For this review, take the finished solid that the model builds, in its own axes (mm). Coordinates: 2 decimals unless noted, no trailing zeros. Write each loop counter-clockwise with the first axis right and the second up, starting at its lowest first coordinate (ties: lowest second). Pieces come first, ordered by that corner, then holes. Notation, with made-up numbers: (29, 1.5) -> (63, 1.5) arc R17 ccw to (63, 10.5) -> close; hole circle Ø9 at (-36, -14.75). An arc over 180 degrees is marked (long way). One line per item, written item: value. Start each with the question number.
1) Add section D-D (z = -62). State the section outline as (x, y) points.
2) Add section C-C (x = -84.5). State the section outline as (y, z) points, and give its area (3 significant figures).
3) Add section B-B (y = 1.2). State how many separate pieces and enclosed holes the cut face has, and give its area (3 significant figures).
4) Add section A-A (x = -40). State the section outline as (y, z) points.
5) For probe 1 along Z at (x, y) = (0, 1.25); probe 2 along Z at (x, y) = (40, 1.1); probe 3 along X at (y, z) = (0.95, 9.5), list the stretches that pass through material, from the lowest coordinate up. Write a range as from..to.
6) Mouldability with a two-part tool opening along X and no side actions: class faces 1 (the flat face through (-78.233, 1.479, -63.383)), 2 (the cylindrical face through (44.995, 1.521, 6.667)), 3 (the flat face through (77.331, 1.479, -64.285)) as released by +X, released by -X, zero draft, split by the parting line, or undercut.
from build123d import *

# Parameters (mm, degrees)
EXTRUDE1_DEPTH     = 3
SKETCH2_R          = 5
CUT_EXTRUDE1_DEPTH = 4
SKETCH7_R          = 5
CUT_EXTRUDE6_DEPTH = 4
SKETCH8_R          = 2.1
CUT_EXTRUDE7_DEPTH = 4


with BuildPart() as part:
    # Sketch1 → Extrude1 (new body)
    with BuildSketch(Plane(origin=(0, 0, 0), x_dir=(1, 0, 0), z_dir=(0, 1, 0))):
        Polygon((-110, -13.947380088), (-110, 31.616111773), (-45.563491861, 96.052619912), (0, 96.052619912), (45.563491861, 96.052619912), (110, 31.616111773), (110, -13.947380088), align=None)
    extrude(amount=EXTRUDE1_DEPTH)

    # Sketch2 → Cut-Extrude1 (cut, through all)
    with BuildSketch(Plane(origin=(0, 3, 0), x_dir=(-1, 0, 0), z_dir=(0, 1, 0))):
        with Locations((85, 6.447380088)):
            Circle(SKETCH2_R)
        with Locations((40, 6.447380088)):
            Circle(SKETCH2_R)
        with Locations((-40, 6.447380088)):
            Circle(SKETCH2_R)
        with Locations((-85, 6.447380088)):
            Circle(SKETCH2_R)
    extrude(amount=-CUT_EXTRUDE1_DEPTH, mode=Mode.SUBTRACT)

    # Sketch7 → Cut-Extrude6 (cut, through all)
    with BuildSketch(Plane(origin=(0, 3, 0), x_dir=(-1, 0, 0), z_dir=(0, 1, 0))):
        with Locations((0, -38.052619912)):
            Circle(SKETCH7_R)
    extrude(amount=-CUT_EXTRUDE6_DEPTH, mode=Mode.SUBTRACT)

    # Sketch8 → Cut-Extrude7 (cut, through all)
    with BuildSketch(Plane(origin=(49.267366711, 3, 2.671437264), x_dir=(-1, 0, 0), z_dir=(0, 1, 0))):
        with Locations((64.267366711, -50.724057176)):
            Circle(SKETCH8_R)
        with Locations((34.267366711, -50.724057176)):
            Circle(SKETCH8_R)
        with Locations((36.277366711, -18.224057176)):
            Circle(SKETCH8_R)
        with Locations((62.257366711, -18.224057176)):
            Circle(SKETCH8_R)
        with Locations((49.267366711, 4.275942824)):
            Circle(SKETCH8_R)
    extrude(amount=-CUT_EXTRUDE7_DEPTH, mode=Mode.SUBTRACT)


solid = part.part
Numbers:
1. outline: (-79.62, 0) -> (79.62, 0) -> (79.62, 3) -> (-79.62, 3) -> close
2. outline: (0, -57.12) -> (3, -57.12) -> (3, 1.47) -> (0, 1.47) -> close; (0, 11.42) -> (3, 11.42) -> (3, 13.95) -> (0, 13.95) -> close
2. area: 183 mm²
3. separate pieces: 1
3. enclosed holes: 10
3. area: 19,600 mm²
4. outline: (0, -96.05) -> (3, -96.05) -> (3, 1.45) -> (0, 1.45) -> close; (0, 11.45) -> (3, 11.45) -> (3, 13.95) -> (0, 13.95) -> close
5. probe 1: -96.05..-43.05, -33.05..4.85, 9.05..13.95
5. probe 2: -96.05..1.45, 11.45..13.95
5. probe 3: -110..-88.96, -81.04..-43.96, -36.04..36.04, 43.96..81.04, 88.96..110
6. face 1: released by -X
6. face 2: undercut
6. face 3: released by +X
